```python
from build123d import *

# Parameters (mm, degrees)
BOSS_EXTRUDE2_DEPTH              = 1.8034
F_97_0_0059_DIAMETER_HOLE1_D     = 4.826
F_13_64_0_20313_DIAMETER_HOLE1_D = 5.159502
SKETCH7_W                        = 29.6164
SKETCH7_H                        = 12.7
CUT_EXTRUDE1_DEPTH               = 2.54


with BuildPart() as part:
    # Sketch1 → Boss-Extrude2 (new body)
    with BuildSketch(Plane.XY):
        Polygon((19.2532, -19.2532), (19.2532, 19.2532), (-19.2532, 19.2532), (-31.9532, 19.2532), (-31.9532, 31.9532), (31.9532, 31.9532), (31.9532, -31.9532), (19.2532, -31.9532), align=None)
    extrude(amount=-BOSS_EXTRUDE2_DEPTH)

    # #97 (0.0059) Diameter Hole1 (through all)
    with Locations(Plane.XY):
        with Locations((-19.3802, 25.6032), (8.4328, 25.6032), (25.6032, -19.3802), (25.6032, 8.4328)):
            Hole(F_97_0_0059_DIAMETER_HOLE1_D / 2)

    # 13/64 (0.20313) Diameter Hole1 (through all)
    with Locations(Plane.XY):
        with Locations((5.6032, 25.6032), (25.6032, 8.4328), (25.6032, -19.3802), (25.6032, 25.6032)):
            Hole(F_13_64_0_20313_DIAMETER_HOLE1_D / 2)

    # Sketch7 → Cut-Extrude1 (cut)
    with BuildSketch(Plane.XY):
        with Locations((-17.145, 25.6032)):
            Rectangle(SKETCH7_W, SKETCH7_H)
    extrude(amount=-CUT_EXTRUDE1_DEPTH, mode=Mode.SUBTRACT)


solid = part.part
```
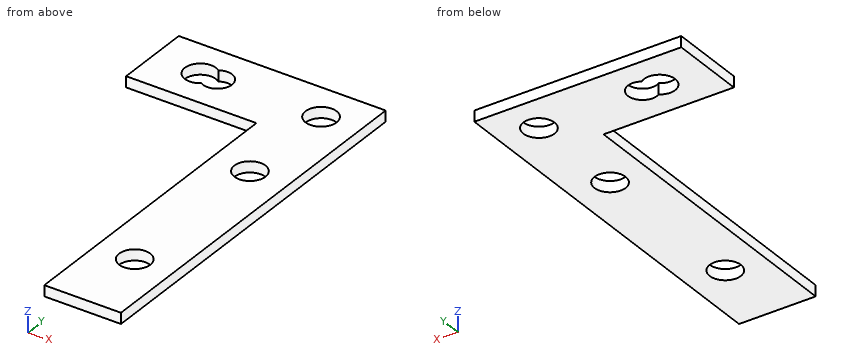
The model under review builds one solid part; all positions refer to its coordinate system, in mm. Round coordinates to 2 decimals unless told otherwise and drop trailing zeros. Write each loop counter-clockwise with the first axis right and the second up, starting at its lowest first coordinate (ties: lowest second). Pieces come first, ordered by that corner, then holes.
(1) We need section B-B on y = -17.5. Give the boundary of the cut face in (x, z), and give its area (3 significant figures).
(2) We need section C-C on y = 26.5. Give the boundary of the cut face in (x, z).
(3) We need section A-A on x = 27. Give the boundary of the cut face in (y, z).
(4) We need section D-D on z = -0.55. Give the boundary of the cut face in (x, y), and give its area (3 significant figures).
(5) Wall thickness on L1, parallel to X at y = -10, z = -0.15; L2, parallel to Y at x = 9, z = -1.55: over which ranges is each line inside the solid? List them lowest first.
(6) Insertion check: pin 1 (0.5 mm diameter, centred on x = 12.5, z = -1, fed in from -Y). The pin has a flat end and moves straight along its axis. Give the tip position at first contact, or say it passes through.
Findings below:
1. outline: (19.25, -1.8) - (23.84, -1.8) - (23.84, 0) - (19.25, 0) - close; (27.37, -1.8) - (31.95, -1.8) - (31.95, 0) - (27.37, 0) - close
1. area: 16.5 mm2
2. outline: (-2.34, -1.8) - (3.18, -1.8) - (3.18, 0) - (-2.34, 0) - close; (10.67, -1.8) - (23.18, -1.8) - (23.18, 0) - (10.67, 0) - close; (28.02, -1.8) - (31.95, -1.8) - (31.95, 0) - (28.02, 0) - close
3. outline: (-31.95, -1.8) - (-21.55, -1.8) - (-21.55, 0) - (-31.95, 0) - close; (-17.21, -1.8) - (6.26, -1.8) - (6.26, 0) - (-17.21, 0) - close; (10.6, -1.8) - (23.43, -1.8) - (23.43, 0) - (10.6, 0) - close; (27.77, -1.8) - (31.95, -1.8) - (31.95, 0) - (27.77, 0) - close
4. outline: (-2.34, 19.25) - (19.25, 19.25) - (19.25, -31.95) - (31.95, -31.95) - (31.95, 31.95) - (-2.34, 31.95) - close; hole (7.17, 23.55) arc R2.41 ccw (long way) to (7.17, 27.66) arc R2.58 ccw (long way) to start; hole circle Ø5.16 at (25.6, -19.38); hole circle Ø5.16 at (25.6, 8.43); hole circle Ø5.16 at (25.6, 25.6)
4. area: 990 mm2
5. L1: x = 19.25 to 31.95
5. L2: y = 19.25 to 23.26, 27.95 to 31.95
6. pin 1: stops at y = 19.25
